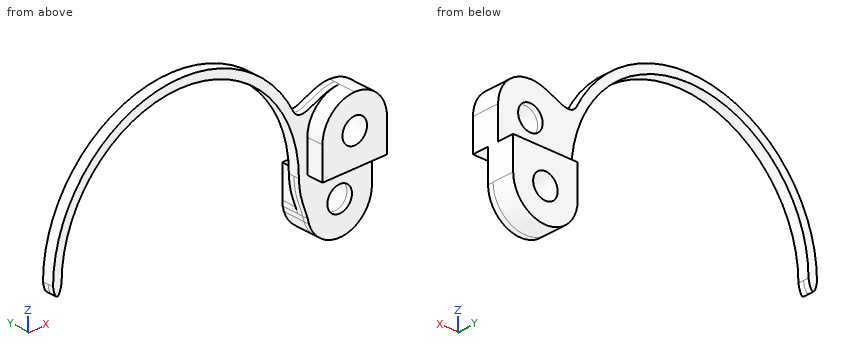
from build123d import *

# Parameters (mm, degrees)
F0_R          = 1.439889
F1_DEPTH      = 2.54
F1_DEPTH_BACK = 0.635
F2_DEPTH      = 0.635
F2_DEPTH_BACK = 2.54
F3_DEPTH      = 0.635
F3_DEPTH_BACK = 0.635


with BuildPart() as f1:
    # F0 (on Front) → F1 (new body, two sides)
    with BuildSketch(Plane.XZ) as f1_sk:
        with BuildLine():
            ThreePointArc((0, 7.488282), (-2.675809, 6.379925), (-3.784166, 3.704116))
            Line((-3.784166, 3.704116), (-3.784166, 0))
            Line((-3.784166, 0), (3.784166, 0))
            Line((3.784166, 0), (3.784166, 3.704116))
            ThreePointArc((3.784166, 3.704116), (2.675809, 6.379925), (0, 7.488282))
        make_face()
        with Locations((0, 3.704116)):
            Circle(F0_R, mode=Mode.SUBTRACT)
    extrude(amount=F1_DEPTH)
    extrude(f1_sk.sketch, amount=-F1_DEPTH_BACK)

    # F0 (on Front) → F2 (join, two sides)
    with BuildSketch(Plane.XZ) as f2_sk:
        with BuildLine():
            Line((3.784166, 0), (-3.784166, 0))
            Line((-3.784166, 0), (-3.784166, -3.704116))
            ThreePointArc((-3.784166, -3.704116), (-3.772481, -4.00126), (-3.7375, -4.296569))
            add(Edge.make_bspline(
                [(-3.7375, -4.296569), (-3.677352, -4.496531), (-3.629914, -4.685815), (-3.601814, -4.864653)],
                knots=[4.234155, 4.234155, 4.234155, 4.234155, 5.005496, 5.005496, 5.005496, 5.005496], degree=3))
            ThreePointArc((-3.601814, -4.864653), (0.587388, -7.442416), (3.784166, -3.704116))
            Line((3.784166, -3.704116), (3.784166, 0))
        make_face()
        with Locations((0, -3.704116)):
            Circle(F0_R, mode=Mode.SUBTRACT)
    extrude(amount=F2_DEPTH)
    extrude(f2_sk.sketch, amount=-F2_DEPTH_BACK)

    # F0 (on Front) → F3 (join, two sides)
    with BuildSketch(Plane.XZ) as f3_sk:
        with BuildLine():
            Line((-3.784166, 0), (-3.784166, 3.704116))
            ThreePointArc((-3.784166, 3.704116), (-2.675809, 6.379925), (0, 7.488282))
            add(Edge.make_bspline(
                [(-5.358132, 6.670184), (-4.27145, 5.197869), (-2.361172, 7.617555), (0, 7.488282)],
                knots=[0, 0, 0, 0, 5.420227, 5.420227, 5.420227, 5.420227], degree=3))
            ThreePointArc((-5.358132, 6.670184), (-4.182987, 3.426687), (-3.784166, 0))
        make_face()
        with BuildLine():
            Line((-3.784166, -3.704116), (-3.784166, 0))
            ThreePointArc((-3.784166, 0), (-4.182987, 3.426687), (-5.358132, 6.670184))
            ThreePointArc((-5.358132, 6.670184), (-22.131354, 14.52168), (-33.62517, 0))
            add(Edge.make_bspline(
                [(-32.628478, 0), (-32.883175, -1.509331), (-33.392582, -1.509331), (-33.62517, 0)],
                knots=[0, 0, 0, 0, 0.996692, 0.996692, 0.996692, 0.996692], degree=3))
            ThreePointArc((-32.628478, 0), (-18.704668, 13.92381), (-4.780858, 0))
            add(Edge.make_bspline(
                [(-4.780858, 0), (-4.780858, -1.779471), (-4.067676, -3.198905), (-3.7375, -4.296569)],
                knots=[0, 0, 0, 0, 4.234155, 4.234155, 4.234155, 4.234155], degree=3))
            ThreePointArc((-3.7375, -4.296569), (-3.772481, -4.00126), (-3.784166, -3.704116))
        make_face()
    extrude(amount=F3_DEPTH)
    extrude(f3_sk.sketch, amount=-F3_DEPTH_BACK)


solid = f1.part
Work out the finished part from the listing and answer in its coordinate system (mm). Give positions to 0.01 mm unless a question says otherwise; leave off trailing zeros. Order: outer loops, then holes, each group sorted by start corner. A loop starts at its lowest first (then second) coordinate and runs counter-clockwise, first axis right, second up. Notation, with made-up numbers: (51.5, 22.5) - (88.5, 22.5) arc R20 cw to (88.5, 32.5) - close; hole circle Ø11 at (13.25, -26.75). An arc over 180 degrees is marked (long way). Answer as CSV lines item,"result". Start each with the question number.
Q1. Find the intervals of material crossed by L1, parallel to X at y = 0.45, z = 4; L2, parallel to X at y = -1.45, z = 3.75; L3, parallel to Z at x = 0, y = -0.75, in increasing order. Write a range as [from, to].
Q2. The part is cut by section D-D (x = -18). Write down the section's boundary in (y, z) (3 decimals).
Q3. The part is cut by section C-C (z = 1.75). Write down the section's boundary in (x, y) (3 decimals).
Q4. The part is cut by section B-B (z = 13). Write down the section's boundary in (x, y) (3 decimals).
Q5. Given pin 1 Ø2 at (x, y) = (-1.5, -2) entering from -Z; pin 2 Ø3 at (x, y) = (-14.5, 1) entering from -Z; pin 3 Ø0.6 at (y, z) = (-1, 2.5) entering from -X, each flat-ended and moving along its own axis, determine where each tip first touches the part or whether it passes through.
Q6. The part is cut by section A-A (y = -1.95). Write down the section's boundary in (x, z).
Check result:
1,L1,"x = [-33.08, -32.04], [-5.37, -1.41], [1.41, 3.77]"
1,L2,"x = [-3.78, -1.44], [1.44, 3.78]"
1,L3,"z = [0, 2.26], [5.14, 7.49]"
2,outline,"(-0.635, 13.906) - (0.635, 13.906) - (0.635, 14.904) - (-0.635, 14.904) - close"
3,outline,"(-33.522, -0.635) - (-32.518, -0.635) - (-32.518, 0.635) - (-33.522, 0.635) - close; (-4.891, -0.635) - (-3.784, -0.635) - (-3.784, -2.54) - (3.784, -2.54) - (3.784, 0.635) - (-4.891, 0.635) - close"
4,outline,"(-26.027, -0.635) - (-23.692, -0.635) - (-23.692, 0.635) - (-26.027, 0.635) - close; (-13.717, -0.635) - (-11.382, -0.635) - (-11.382, 0.635) - (-13.717, 0.635) - close"
5,pin 1,"stops at z = 0"
5,pin 2,"stops at z = 12.72"
5,pin 3,"stops at x = -3.78"
6,outline,"(-3.78, 0) - (3.78, 0) - (3.78, 3.7) arc R3.78 ccw to (0, 7.49) arc R3.78 ccw to (-3.78, 3.7) - close; hole circle Ø2.88 at (0, 3.7)"
